Model file for the job. Use its own axes, mm. Face numbers are marked on the shaded views. A direction names the side the tool comes from. Round coordinates to 2 decimals unless told otherwise and drop trailing zeros. Loops run counter-clockwise (first coordinate to the right, second up) from the corner with the lowest first, then second, coordinate; pieces in that order, holes last. Notation, with made-up numbers: (-3, 44.5) - (34, 44.5) arc R25 cw to (34, 67.5) - close; hole circle Ø10 at (-25.5, 23). An arc over 180 degrees is marked (long way). Use one line per item in the form item = value.
from build123d import *

# Parameters (mm, degrees)
SKETCH1_W               = 90
SKETCH1_H               = 35
BOSS_EXTRUDE1_DEPTH     = 60
SKETCH2_W               = 25
SKETCH2_H               = 13
CUT_EXTRUDE1_DEPTH      = 8
SKETCH3_R               = 14.5
CUT_EXTRUDE2_DEPTH      = 96.131487952
CUT_EXTRUDE8_DEPTH      = 110.676797911
CUT_EXTRUDE8_DEPTH_BACK = 2
SKETCH4_W               = 95.939068785
SKETCH4_H               = 13


with BuildPart() as part:
    # Sketch1 → Boss-Extrude1 (new body)
    with BuildSketch(Plane(origin=(0, 0, 0), x_dir=(1, 0, 0), z_dir=(0, 1, 0))):
        with Locations((45, -17.5)):
            Rectangle(SKETCH1_W, SKETCH1_H)
    extrude(amount=BOSS_EXTRUDE1_DEPTH)

    # Sketch2 → Cut-Extrude1 (cut)
    with BuildSketch(Plane(origin=(0, 60, 0), x_dir=(1, 0, 0), z_dir=(0, 1, 0))):
        with Locations((77.5, -17.5)):
            Rectangle(SKETCH2_W, SKETCH2_H)
    extrude(amount=-CUT_EXTRUDE1_DEPTH, mode=Mode.SUBTRACT)

    # Sketch3 → Cut-Extrude2 (cut, through all)
    with BuildSketch(Plane(origin=(65, 0, 0), x_dir=(0, 0, -1), z_dir=(1, 0, 0))):
        with Locations((-17.5, 66.5)):
            Circle(SKETCH3_R)
    extrude(amount=-CUT_EXTRUDE2_DEPTH, mode=Mode.SUBTRACT)

    # Sketch4 → Cut-Extrude8 (cut, two sides: drawn at the far end of the back side and taken through both)
    with BuildSketch(Plane(origin=(0, 52, 0), x_dir=(1, 0, 0), z_dir=(0, 1, 0)).offset(-CUT_EXTRUDE8_DEPTH_BACK)):
        with Locations((42.030465607, -17.5)):
            Rectangle(SKETCH4_W, SKETCH4_H)
    extrude(amount=CUT_EXTRUDE8_DEPTH + CUT_EXTRUDE8_DEPTH_BACK, mode=Mode.SUBTRACT)


solid = part.part
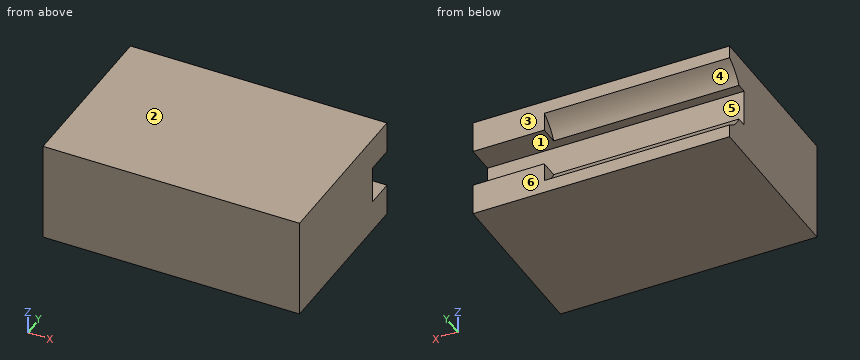
1. Cut at B-B, the plane z = 8. Give the cut face in (x, y), plus the area to 3 significant figures.
Geometry check:
outline = (0, 0) - (90, 0) - (90, 60) - (65, 60) - (65, 55.55) - (0, 55.55) - close
area = 5,110 mm^2
2. Wall check: probe 1 along Z at (x, y) = (18, 53); probe 2 along Y at (x, z) = (15, 23); probe 3 along Y at (x, z) = (36, 10). Give the ranges that are in metal, low to high.
Geometry check:
probe_1 = 0 to 11, 24 to 35
probe_2 = 0 to 50
probe_3 = 0 to 54.09
3. Flat gauge pins, fed straight in: pin 1 (6.5 mm diameter, centred on x = 60, z = 18.5, fed in from +Y); pin 2 (5 mm diameter, centred on x = 55, y = 55, fed in from -Z). Where does each tip first touch, or does it go through?
Geometry check:
pin_1 = 50
pin_2 = 0
4. Pull direction Z, two halves, no side cores. Call the marked faces 1, 2 and 3: +Z half, -Z half, draft (parallel to the pull), parting line (faces both ways), or undercut.
Geometry check:
face_1 = undercut
face_2 = +Z half
face_3 = draft
5. Tool access for the marked faces 4, 5 and 6: list every direction of +Z, -Z, +X, -X, +Y, -Y with a clear straight run to the whole face (end or side of a thin tool).
Geometry check:
face_4 = -X, +Y
face_5 = +X, -X, +Y
face_6 = +Z, -Z, +X, -X, +Y
6. Cut at A-A, the plane x = 67.5. Give the cut face in (y, z), plus the area to 3 significant figures.
Geometry check:
outline = (0, 0) - (60, 0) - (60, 11) - (50, 11) - (50, 24) - (60, 24) - (60, 35) - (0, 35) - close
area = 1,970 mm^2
7. Cut at C-C, the plane x = 49.5. Give the cut face in (y, z), plus the area to 3 significant figures.
Geometry check:
outline = (0, 0) - (60, 0) - (60, 4.54) arc R14.5 cw to (53.54, 11) - (50, 11) - (50, 24) - (53.54, 24) arc R14.5 cw to (60, 30.46) - (60, 35) - (0, 35) - close
area = 1,920 mm^2
